```python
from build123d import *

# Parameters (mm, degrees)
SKIZZE1_W                                   = 300
SKIZZE1_H                                   = 234
AUFSATZ_LINEAR_AUSTRAGEN1_DEPTH             = 4
VERRUNDUNG1_R                               = 17
FORMSENKUNG_F_R_M6_SENKSCHRAUBE_MIT_2_COUNT = 2
FORMSENKUNG_F_R_M6_SENKSCHRAUBE_MIT_2_PITCH = 280
FORMSENKUNG_F_R_M6_SENKSCHRAUBE_MIT_3_COUNT = 2
FORMSENKUNG_F_R_M6_SENKSCHRAUBE_MIT_3_PITCH = 362.35341864
FORMSENKUNG_F_R_M6_SENKSCHRAUBE_MIT_4_COUNT = 2
FORMSENKUNG_F_R_M6_SENKSCHRAUBE_MIT_4_PITCH = 230


with BuildPart() as part:
    # Skizze1 → Aufsatz-Linear austragen1 (new body)
    with BuildSketch(Plane(origin=(0, 0, 0), x_dir=(1, 0, 0), z_dir=(0, 1, 0))):
        with Locations((150, 117)):
            Rectangle(SKIZZE1_W, SKIZZE1_H)
    extrude(amount=AUFSATZ_LINEAR_AUSTRAGEN1_DEPTH)

    # Verrundung1
    verrundung1_edges = [part.edges().sort_by_distance(p)[0] for p in [
        (300, 2, 0),
        (0, 2, 0),
    ]]
    fillet(verrundung1_edges, radius=VERRUNDUNG1_R)

    # Skizze2 → Formsenkung für M6 Senkschraube mit Schlitz/Kreuzschlitz1 (revolve, cut)
    with BuildSketch(Plane(origin=(10, 4, -10), x_dir=(0, 0, 1), z_dir=(1, 0, 0))):
        Polygon((0, 0), (0, 4), (3.2, 4), (3.2, 3.1), (6.3, 0), align=None)
    formsenkung_f_r_m6_senkschraube_mit_schl = revolve(axis=Axis((10, 10.35, -10), (0, -1, 0)), mode=Mode.SUBTRACT)

    # Formsenkung f_r M6 Senkschraube mit  2: Formsenkung für M6 Senkschraube mit Schlitz/Kreuzschlitz1 ×2
    with Locations(*[(i * FORMSENKUNG_F_R_M6_SENKSCHRAUBE_MIT_2_PITCH, 0, 0) for i in range(1, FORMSENKUNG_F_R_M6_SENKSCHRAUBE_MIT_2_COUNT)]):
        add(formsenkung_f_r_m6_senkschraube_mit_schl, mode=Mode.SUBTRACT)

    # Formsenkung f_r M6 Senkschraube mit  3: Formsenkung für M6 Senkschraube mit Schlitz/Kreuzschlitz1 ×2
    with Locations(*[Vector(0.7727262545252342, 0, -0.6347394233600139) * (i * FORMSENKUNG_F_R_M6_SENKSCHRAUBE_MIT_3_PITCH) for i in range(1, FORMSENKUNG_F_R_M6_SENKSCHRAUBE_MIT_3_COUNT)]):
        add(formsenkung_f_r_m6_senkschraube_mit_schl, mode=Mode.SUBTRACT)

    # Formsenkung f_r M6 Senkschraube mit  4: Formsenkung für M6 Senkschraube mit Schlitz/Kreuzschlitz1 ×2
    with Locations(*[(0, 0, -i * FORMSENKUNG_F_R_M6_SENKSCHRAUBE_MIT_4_PITCH) for i in range(1, FORMSENKUNG_F_R_M6_SENKSCHRAUBE_MIT_4_COUNT)]):
        add(formsenkung_f_r_m6_senkschraube_mit_schl, mode=Mode.SUBTRACT)


solid = part.part
```
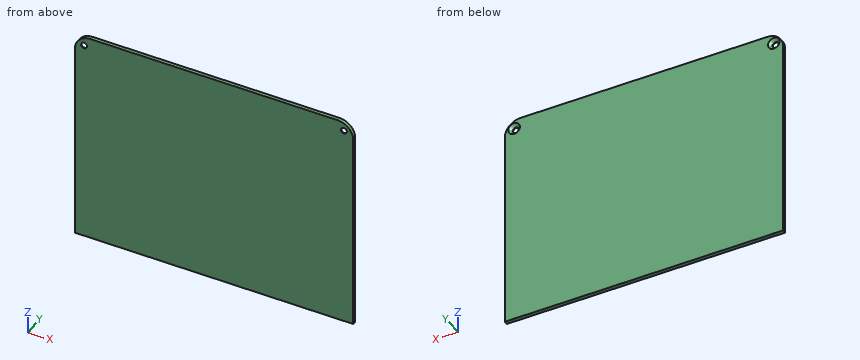
Check sheet for the modelled part. Datum: model origin and axes. Units: mm. Coordinates: 2 decimals unless noted, no trailing zeros. Write each loop counter-clockwise with the first axis right and the second up, starting at its lowest first coordinate (ties: lowest second). Pieces come first, ordered by that corner, then holes. Notation, with made-up numbers: (62.25, -27) -> (78.25, -27) arc R21 cw to (78.25, 4) -> close; hole circle Ø3 at (-32, 9.25). An arc over 180 degrees is marked (long way). Use a Markdown table: item, result.
1. Scan lines: line 1 along X through (y, z) = (0.5, -10); line 2 along Z through (x, y) = (290, 0.55); line 3 along X through (y, z) = (2.9, -10.5). Record each from-to range of solid material in increasing order.
Reported:
| item | result |
|---|---|
| line 1 | x = 1.51 to 6.8, 13.2 to 286.8, 293.2 to 298.49 |
| line 2 | z = -234 to -13.2, -6.8 to -1.51 |
| line 3 | x = 1.29 to 4.82, 15.18 to 284.82, 295.18 to 298.71 |
2. Sectioned sample at A-A (z = -10). Enter the section's corners in (x, y).
Reported:
| item | result |
|---|---|
| outline | (1.51, 0) -> (6.8, 0) -> (6.8, 0.9) -> (3.7, 4) -> (1.51, 4) -> close; (13.2, 0) -> (286.8, 0) -> (286.8, 0.9) -> (283.7, 4) -> (16.3, 4) -> (13.2, 0.9) -> close; (293.2, 0) -> (298.49, 0) -> (298.49, 4) -> (296.3, 4) -> (293.2, 0.9) -> close |
3. Go/stop test with flat-tipped pins: pin 1 Ø4 at (x, z) = (290, -10) entering from -Y; pin 2 Ø8 at (x, z) = (147.5, -26.5) entering from -Y; pin 3 Ø8.5 at (x, z) = (10, -10) entering from +Y. Record where each tip stops, or that it passes through.
Reported:
| item | result |
|---|---|
| pin 1 | passes through |
| pin 2 | stops at y = 0 |
| pin 3 | stops at y = 1.95 |
